The figure shows three views and two pictorial views of one solid part (mm, origin at its lowest corner). Answer the questions. A direction names the side the tool comes from. Round coordinates to 2 decimals unless told otherwise and drop trailing zeros. Order: outer loops, then holes, each group sorted by start corner. A loop starts at its lowest first (then second) coordinate and runs counter-clockwise, first axis right, second up. Notation, with made-up numbers: (35, 25.25) -> (70, 25.25) arc R25 cw to (70, 45.25) -> close; hole circle Ø8 at (-11, -36.75). An arc over 180 degrees is marked (long way). One line per item, written item: value. Start each with the question number.
1. Section D-D (z = 53) is taken. Give the vertices of the cut face in (x, y).
2. The mould has two halves that part along Y. Classify the marked faces 6, 7 and 8: released by +Y, released by -Y, zero draft, split by the parting line, or undercut.
3. For the marked faces 1, 2, 3, 4 and 5, determine the directions among +Z, -Z, +X, -X, +Y, -Y from which every point of the face is accessible in a straight line to the end or side of a thin tool.
4. Section C-C (x = 48) is taken. Give the vertices of the cut face in (y, z), then the cut area to 3 significant figures.
5. Section B-B (y = 13.5) is taken. Give the vertices of the cut face in (x, z).
6. Consider line 1 (Y direction, x = 22, z = 37); line 2 (X direction, y = 31.5, z = 21); line 3 (X direction, y = 23, z = 46.5). Determine where each line is inside the solid, lowest interval first.
7. Section A-A (z = 9) is taken. Give the vertices of the cut face in (x, y).
8. Flat-ended cylindrical pins translate along their axes: pin 1 Ø4 at (y, z) = (23, 56.5) entering from -X; pin 2 Ø2 at (x, z) = (38.5, 39) entering from -Y; pin 3 Ø2 at (y, z) = (1.5, 34.5) entering from +X; pin 4 Ø1.5 at (y, z) = (10.5, 13.5) entering from -X. Find the tip coordinate at first contact, or state that the pin passes through.
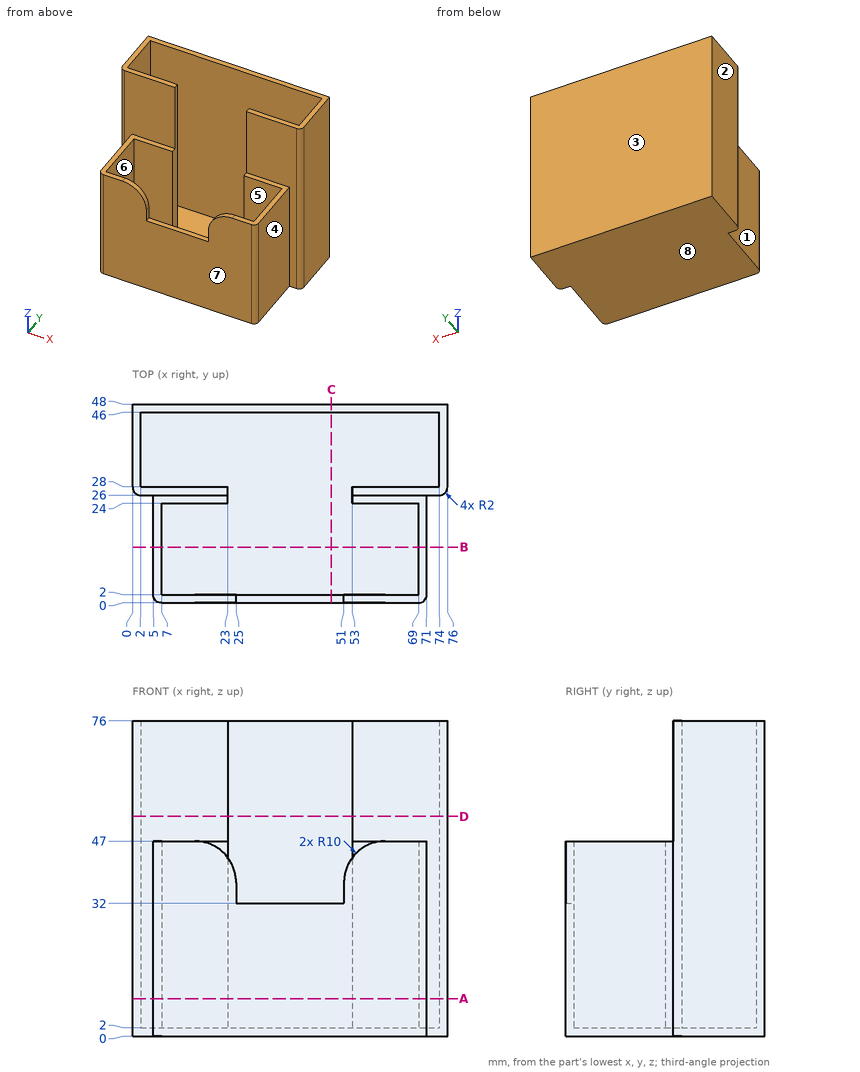
Answer:
1. outline: (0, 28) arc R2 ccw to (2, 26) -> (23, 26) -> (23, 28) -> (2, 28) -> (2, 46) -> (74, 46) -> (74, 28) -> (53, 28) -> (53, 26) -> (74, 26) arc R2 ccw to (76, 28) -> (76, 48) -> (0, 48) -> close
2. face 6: undercut
2. face 7: released by -Y
2. face 8: zero draft
3. face 1: +Z, -Z, -X, -Y
3. face 2: +Z, -Z, -X, +Y, -Y
3. face 3: +Z, -Z, +X, -X, +Y
3. face 4: +Z, -Z, +X, -Y
3. face 5: +Z
4. outline: (0, 0) -> (48, 0) -> (48, 76) -> (46, 76) -> (46, 2) -> (2, 2) -> (2, 32) -> (0, 32) -> close
4. area: 304 mm^2
5. outline: (5, 0) -> (71, 0) -> (71, 47) -> (69, 47) -> (69, 2) -> (7, 2) -> (7, 47) -> (5, 47) -> close
6. line 1: 0 to 2, 24 to 28, 46 to 48
6. line 2: 0 to 2, 74 to 76
6. line 3: 5 to 7, 69 to 71
7. outline: (0, 28) arc R2 ccw to (2, 26) -> (5, 26) -> (5, 2) arc R2 ccw to (7, 0) -> (69, 0) arc R2 ccw to (71, 2) -> (71, 26) -> (74, 26) arc R2 ccw to (76, 28) -> (76, 48) -> (0, 48) -> close; hole (2, 28) -> (23, 28) -> (23, 24) -> (7, 24) -> (7, 2) -> (69, 2) -> (69, 24) -> (53, 24) -> (53, 28) -> (74, 28) -> (74, 46) -> (2, 46) -> close
8. pin 1: through
8. pin 2: y = 46
8. pin 3: x = 71
8. pin 4: x = 5
